```python
from build123d import *

# Parameters (mm, degrees)
CROQUIS1_W              = 45
CROQUIS1_H              = 20
SALIENTE_EXTRUIR1_DEPTH = 2
CROQUIS2_R              = 8
SALIENTE_EXTRUIR2_DEPTH = 12
REDONDEO1_R             = 1
SALIENTE_EXTRUIR3_DEPTH = 3
REDONDEO2_R             = 1
CROQUIS4_R              = 0.5
CORTAR_EXTRUIR1_DEPTH   = 3
CROQUIS5_W              = 10
CROQUIS5_H              = 3
SALIENTE_EXTRUIR4_DEPTH = 2.54
CHAFL_N1_SIZE           = 0.2
CROQUIS6_W              = 0.7
CROQUIS6_H              = 0.7
SALIENTE_EXTRUIR5_DEPTH = 1
CROQUIS7_W              = 0.7
CROQUIS7_H              = 0.7
REVOLUCI_N1_ANGLE       = 90
CROQUIS8_W              = 0.7
CROQUIS8_H              = 0.7
SALIENTE_EXTRUIR6_DEPTH = 6


with BuildPart() as part:
    # Croquis1 → Saliente-Extruir1 (new body)
    with BuildSketch(Plane.XY):
        Rectangle(CROQUIS1_W, CROQUIS1_H)
    extrude(amount=SALIENTE_EXTRUIR1_DEPTH)

    # Croquis2 → Saliente-Extruir2 (add)
    with BuildSketch(Plane.XY.offset(2)):
        with Locations((12.5, 0)):
            Circle(CROQUIS2_R)
        with Locations((-12.5, 0)):
            Circle(CROQUIS2_R)
    extrude(amount=SALIENTE_EXTRUIR2_DEPTH)

    # Redondeo1
    redondeo1_edges = [part.edges().sort_by_distance(p)[0] for p in [
        (4.5, 0, 2),
        (4.5, 0, 14),
        (-20.5, 0, 2),
        (-20.5, 0, 14),
    ]]
    fillet(redondeo1_edges, radius=REDONDEO1_R)

    # Croquis3 → Saliente-Extruir3 (add)
    with BuildSketch(Plane.XY.offset(2)):
        with BuildLine():
            Line((4, 5.5), (-4, 5.5))
            ThreePointArc((-4, 5.5), (-5.75, 7.25), (-4, 9))
            Line((-4, 9), (4, 9))
            ThreePointArc((4, 9), (5.75, 7.25), (4, 5.5))
        make_face()
    extrude(amount=SALIENTE_EXTRUIR3_DEPTH)

    # Redondeo2
    redondeo2_edges = [part.edges().sort_by_distance(p)[0] for p in [
        (5.75, 7.25, 5),
        (0, 9, 5),
        (-5.75, 7.25, 5),
        (0, 5.5, 5),
    ]]
    fillet(redondeo2_edges, radius=REDONDEO2_R)

    # Croquis4 → Cortar-Extruir1 (cut, through all)
    with BuildSketch(Plane.XY.offset(2)):
        with Locations((21.5, 9)):
            Circle(CROQUIS4_R)
        with Locations((21.5, -9)):
            Circle(CROQUIS4_R)
        with Locations((-21.5, -9)):
            Circle(CROQUIS4_R)
        with Locations((-21.5, 9)):
            Circle(CROQUIS4_R)
    extrude(amount=-CORTAR_EXTRUIR1_DEPTH, mode=Mode.SUBTRACT)

    # Croquis5 → Saliente-Extruir4 (add)
    with BuildSketch(Plane(origin=(0, 0, 0), x_dir=(-1, 0, 0), z_dir=(0, 0, -1))):
        with Locations((0, -8.5)):
            Rectangle(CROQUIS5_W, CROQUIS5_H)
    extrude(amount=SALIENTE_EXTRUIR4_DEPTH)

    # Chaflán1
    chafl_n1_edges = [part.edges().sort_by_distance(p)[0] for p in [
        (5, -7, -1.27),
        (5, -10, -1.27),
        (-5, -10, -1.27),
        (-5, -7, -1.27),
    ]]
    chamfer(chafl_n1_edges, length=CHAFL_N1_SIZE)

    # Croquis6 → Saliente-Extruir5 (add)
    with BuildSketch(Plane(origin=(0, 0, -2.54), x_dir=(-1, 0, 0), z_dir=(0, 0, -1))):
        with Locations((-3.75, -8.5)):
            Rectangle(CROQUIS6_W, CROQUIS6_H)
        with Locations((-1.25, -8.5)):
            Rectangle(CROQUIS6_W, CROQUIS6_H)
        with Locations((1.25, -8.5)):
            Rectangle(CROQUIS6_W, CROQUIS6_H)
        with Locations((3.75, -8.5)):
            Rectangle(CROQUIS6_W, CROQUIS6_H)
    extrude(amount=SALIENTE_EXTRUIR5_DEPTH)

    # Croquis7 → Revolución1 (revolve)
    with BuildSketch(Plane(origin=(0, 0, -3.54), x_dir=(-1, 0, 0), z_dir=(0, 0, -1))):
        with Locations((-3.75, -8.5)):
            Rectangle(CROQUIS7_W, CROQUIS7_H)
        with Locations((-1.25, -8.5)):
            Rectangle(CROQUIS7_W, CROQUIS7_H)
        with Locations((1.25, -8.5)):
            Rectangle(CROQUIS7_W, CROQUIS7_H)
        with Locations((3.75, -8.5)):
            Rectangle(CROQUIS7_W, CROQUIS7_H)
    revolve(axis=Axis((4.1, -9.15, -3.54), (-1, 0, 0)), revolution_arc=REVOLUCI_N1_ANGLE)

    # Croquis8 → Saliente-Extruir6 (add)
    with BuildSketch(Plane.XZ.offset(9.15)):
        with Locations((3.75, -4.19)):
            Rectangle(CROQUIS8_W, CROQUIS8_H)
        with Locations((1.25, -4.19)):
            Rectangle(CROQUIS8_W, CROQUIS8_H)
        with Locations((-1.25, -4.19)):
            Rectangle(CROQUIS8_W, CROQUIS8_H)
        with Locations((-3.75, -4.19)):
            Rectangle(CROQUIS8_W, CROQUIS8_H)
    extrude(amount=SALIENTE_EXTRUIR6_DEPTH)


solid = part.part
```
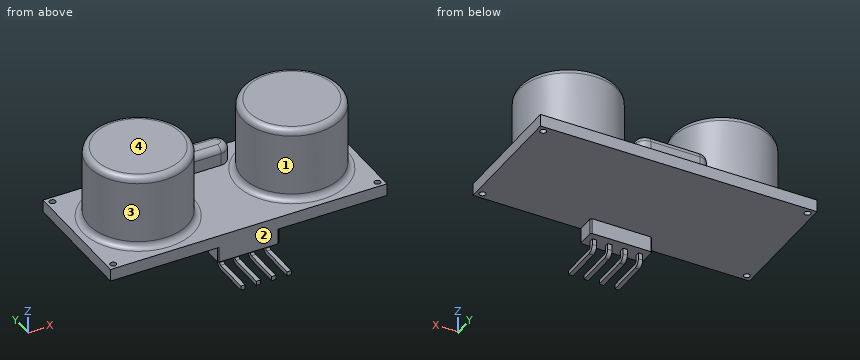
Check sheet for the modelled part. Datum: model origin and axes. Units: mm. Face numbers are marked on the shaded views. A direction names the side the tool comes from. Coordinates: 2 decimals unless noted, no trailing zeros. Order: outer loops, then holes, each group sorted by start corner. A loop starts at its lowest first (then second) coordinate and runs counter-clockwise, first axis right, second up. Notation, with made-up numbers: M 26,42.25 L 67,42.25 A22 ccw 67,54.25 Z; hole C -4,71.5 d8. An arc over 180 degrees is marked long. Write each question's results on one line, items separated by ' | '. Start each with the question number.
1. Cross-section at B-B on y = -12. Record the cut outline in (x, z).
2. Cross-section at D-D on z = 11.5. Record the cut outline in (x, y).
3. Cross-section at C-C on x = 0. Record the cut outline in (y, z), and give its area (3 significant figures).
4. Access from +Z, -Z, +X, -X, +Y, -Y to the whole of each face (thin tool, end or side, straight path). Record for the marked faces 3 and 4.
5. Cross-section at A-A on z = 3.5. Record the cut outline in (x, y).
6. Mould release check, pull along X, two halves, no side actions. Record for the marked faces 1 and 2: +X half, -X half, draft (parallel to the pull), parting line (faces both ways), or undercut.
7. Material ranges on probe 1 along Y at (x, z) = (21.5, 0.9); probe 2 along Z at (x, y) = (19, 9); probe 3 along Y at (x, z) = (4, 2.25), recorded low to high.
8. Go/stop test with flat-tipped pins: P1, Ø1.3, axis at x = -0.5, z = -1.5, coming from the +Y side; P2, Ø10, axis at x = -6.5, y = -3.5, coming from the -Z side; P3, Ø0.8, axis at x = -1.5, z = -3, coming from the +Y side; P4, Ø0.6, axis at y = -11, z = -3.5, coming from the -X side. Record where each tip stops, or that it passes through.
Checks:
1) outline: M -4.1,-4.54 L -3.4,-4.54 L -3.4,-3.84 L -4.1,-3.84 Z; M -1.6,-4.54 L -0.9,-4.54 L -0.9,-3.84 L -1.6,-3.84 Z; M 0.9,-4.54 L 1.6,-4.54 L 1.6,-3.84 L 0.9,-3.84 Z; M 3.4,-4.54 L 4.1,-4.54 L 4.1,-3.84 L 3.4,-3.84 Z
2) outline: C -12.5,0 d16; C 12.5,0 d16
3) outline: M -10,-2.54 L -7,-2.54 L -7,0 L 10,0 L 10,2 L 9,2 L 9,4 A1 ccw 8,5 L 6.5,5 A1 ccw 5.5,4 L 5.5,2 L -10,2 Z | area: 57.7 mm²
4) face 3: +Z | face 4: +Z, +X, -X, +Y, -Y
5) outline: C -12.5,0 d16; M -4,5.5 L 4,5.5 A1.75 ccw 4,9 L -4,9 A1.75 ccw Z; C 12.5,0 d16
6) face 1: undercut | face 2: draft
7) probe 1: y = -10 to -9.5, -8.5 to 8.5, 9.5 to 10 | probe 2: z = 0 to 2 | probe 3: y = 5.5 to 9
8) P1: stops at y = -7 | P2: stops at z = -2.54 | P3: stops at y = -8.15 | P4: passes through
